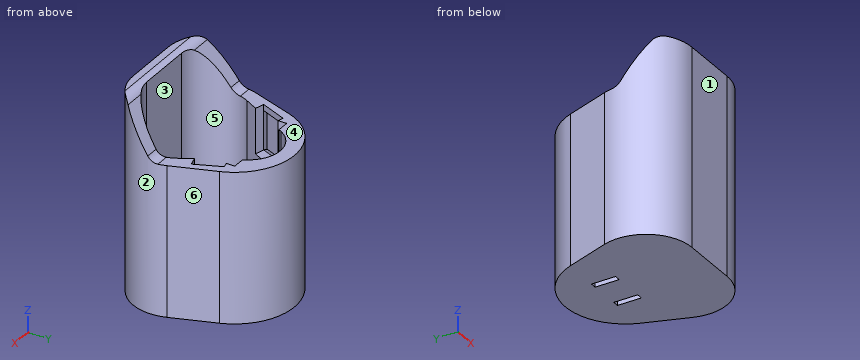
from build123d import *

# Parameters (mm, degrees)
RESSALTO_EXTRUS_O1_DEPTH   = 66
CORTE_EXTRUS_O1_DEPTH      = 53.5
CORTE_EXTRUS_O2_DEPTH      = 9.5
ESBO_O5_W                  = 2
ESBO_O5_H                  = 8
CORTE_EXTRUS_O3_DEPTH      = 72.859720289
CORTE_EXTRUS_O4_DEPTH      = 75.503821379
CORTE_EXTRUS_O4_DEPTH_BACK = 75.503821379
CORTE_EXTRUS_O6_DEPTH      = 15
ESBO_O10_W                 = 13
ESBO_O10_H                 = 9.498093923
CORTE_EXTRUS_O7_DEPTH      = 1.8
CORTE_EXTRUS_O7_DRAFT      = 23
ESBO_O11_W                 = 13
ESBO_O11_H                 = 9.498093923
CORTE_EXTRUS_O8_DEPTH      = 1.8
CORTE_EXTRUS_O8_DRAFT      = 23
FILETE10_START             = -24.75
FILETE10_DEPTH             = 49.5
FILETE11_R                 = 4
FILETE12_R                 = 4
CORTE_EXTRUS_O9_DEPTH      = 47


with BuildPart() as part:
    # Esboço2 → Ressalto-extrusão1 (new body)
    with BuildSketch(Plane.XY):
        with BuildLine():
            Line((18.875125561, 10.742838653), (23.89228324, -3.577710527))
            ThreePointArc((23.89228324, -3.577710527), (21.938999447, -17.442346217), (9.5, -23.87))
            Line((9.5, -23.87), (-9.5, -23.87))
            ThreePointArc((-9.5, -23.87), (-21.938999447, -17.442346217), (-23.89228324, -3.577710527))
            Line((-23.89228324, -3.577710527), (-18.875125561, 10.742838653))
            ThreePointArc((-18.875125561, 10.742838653), (0, 24.13), (18.875125561, 10.742838653))
        make_face()
    extrude(amount=RESSALTO_EXTRUS_O1_DEPTH)

    # Esboço3 → Corte-extrusão1 (cut)
    with BuildSketch(Plane.XY.offset(66)):
        with BuildLine():
            Line((-9.315367954, 13.892017036), (-18.902836198, -3.409513321))
            ThreePointArc((-18.902836198, -3.409513321), (-18.762160434, -14.076636702), (-9.5, -19.37))
            Line((-9.5, -19.37), (9.5, -19.37))
            ThreePointArc((9.5, -19.37), (18.762160434, -14.076636702), (18.902836198, -3.409513321))
            Line((18.902836198, -3.409513321), (9.315367954, 13.892017036))
            ThreePointArc((9.315367954, 13.892017036), (0, 19.38), (-9.315367954, 13.892017036))
        make_face()
    extrude(amount=-CORTE_EXTRUS_O1_DEPTH, mode=Mode.SUBTRACT)

    # Esboço4 → Corte-extrusão2 (cut)
    with BuildSketch(Plane.XY.offset(12.5)):
        with BuildLine():
            Line((-9.315367954, 13.892017036), (-18.88094029, -3.37))
            Line((-18.88094029, -3.37), (18.88094029, -3.37))
            Line((18.88094029, -3.37), (9.315367954, 13.892017036))
            ThreePointArc((9.315367954, 13.892017036), (0, 19.38), (-9.315367954, 13.892017036))
        make_face()
    extrude(amount=-CORTE_EXTRUS_O2_DEPTH, mode=Mode.SUBTRACT)

    # Esboço5 → Corte-extrusão3 (cut, through all)
    with BuildSketch(Plane.XY.offset(3)):
        with Locations((-6, 7.13)):
            Rectangle(ESBO_O5_W, ESBO_O5_H)
        with Locations((6, 7.13)):
            Rectangle(ESBO_O5_W, ESBO_O5_H)
    extrude(amount=-CORTE_EXTRUS_O3_DEPTH, mode=Mode.SUBTRACT)

    # Esboço6 → Corte-extrusão4 (cut, two sides: drawn at the far end of the back side and taken through both)
    with BuildSketch(Plane(origin=(0, 0, 0), x_dir=(0, 0, -1), z_dir=(1, 0, 0)).offset(-CORTE_EXTRUS_O4_DEPTH_BACK)):
        Polygon((-73.252948894, -8.37), (-72.738467135, 18.869608141), (-69.396784042, 24.687681426), (-65.169347817, 25.830591912), (-50, 27.529066054), (-50, -8.37), (-66, -19.37), (-66, -23.87), (-79.476934269, -23.87), (-79.476934269, -8.37), align=None)
    extrude(amount=CORTE_EXTRUS_O4_DEPTH + CORTE_EXTRUS_O4_DEPTH_BACK, mode=Mode.SUBTRACT)

    # Esboço7 → Corte-extrusão6 (cut)
    with BuildSketch(Plane.XY.offset(50)):
        Polygon((0, -3.37), (19.549187838, 1.7499651), (15.86238212, 10.5033217), (2e-09, 6.348937203), (-15.862382121, 10.5033217), (-19.549187841, 1.7499651), align=None)
    extrude(amount=-CORTE_EXTRUS_O6_DEPTH, mode=Mode.SUBTRACT)


with BuildPart() as corte_extrus_o7_tool:
    # Esboço10 → Corte-extrusão7 (with draft: the straight prism first)
    with BuildSketch(Plane(origin=(17.229716404, 7.256943806, 0), x_dir=(0, 0, 1), z_dir=(-0.9215908655875538, -0.3881626932944273, 0))):
        with Locations((41.5, -1.226466591)):
            Rectangle(ESBO_O10_W, ESBO_O10_H)
    extrude(amount=-CORTE_EXTRUS_O7_DEPTH)
    # Corte-extrusão7: the draft: its side faces are tilted about the plane it starts from
    corte_extrus_o7_sides = [corte_extrus_o7_tool.faces().sort_by_distance(p)[0] for p in [
        (16.691813899, 10.852668124, 41.5),
        (18.535216758, 6.475989824, 35),
        (20.378619617, 2.099311524, 41.5),
        (18.535216758, 6.475989824, 48),
    ]]
    draft(corte_extrus_o7_sides, Plane(origin=(17.229716404, 7.256943806, 0), x_dir=(0, 0, 1), z_dir=(-0.9215908655875538, -0.3881626932944273, 0)), CORTE_EXTRUS_O7_DRAFT)


with BuildPart() as part_1:
    add(part.part)

    # Corte-extrusão7: cut by corte_extrus_o7_tool
    add(corte_extrus_o7_tool.part, mode=Mode.SUBTRACT)


with BuildPart() as corte_extrus_o8_tool:
    # Esboço11 → Corte-extrusão8 (with draft: the straight prism first)
    with BuildSketch(Plane(origin=(-17.229716404, 7.256943809, 0), x_dir=(0, 0, -1), z_dir=(0.9215908655337633, -0.3881626934221387, 0))):
        with Locations((-41.5, -1.226466593)):
            Rectangle(ESBO_O11_W, ESBO_O11_H)
    extrude(amount=-CORTE_EXTRUS_O8_DEPTH)
    # Corte-extrusão8: the draft: its side faces are tilted about the plane it starts from
    corte_extrus_o8_sides = [corte_extrus_o8_tool.faces().sort_by_distance(p)[0] for p in [
        (-18.53521676, 6.475989824, 48),
        (-20.37861962, 2.099311524, 41.5),
        (-18.53521676, 6.475989824, 35),
        (-16.6918139, 10.852668124, 41.5),
    ]]
    draft(corte_extrus_o8_sides, Plane(origin=(-17.229716404, 7.256943809, 0), x_dir=(0, 0, -1), z_dir=(0.9215908655337633, -0.3881626934221387, 0)), CORTE_EXTRUS_O8_DRAFT)


with BuildPart() as part_2:
    add(part_1.part)

    # Corte-extrusão8: cut by corte_extrus_o8_tool
    add(corte_extrus_o8_tool.part, mode=Mode.SUBTRACT)

    # Filete10: read off the stored shape, not the designer's step
    # Filete10 outline → Filete10 (cut)
    with BuildSketch(Plane.YZ.offset(FILETE10_START)):
        with BuildLine():
            ThreePointArc((-21.47412196, 66), (-19.611926245, 65.540088576), (-18.177953073, 64.266113561))
            Line((-18.177953073, 64.266113561), (-19.37, 66))
            Line((-19.37, 66), (-21.47412196, 66))
        make_face()
    extrude(amount=FILETE10_DEPTH, mode=Mode.SUBTRACT)

    # Filete11
    filete11_edges = [part_2.edges().sort_by_distance(p)[0] for p in [
        (-22.497521656, -8.37, 50),
    ]]
    fillet(filete11_edges, radius=FILETE11_R)

    # Filete12
    filete12_edges = [part_2.edges().sort_by_distance(p)[0] for p in [
        (22.497521656, -8.37, 50),
    ]]
    fillet(filete12_edges, radius=FILETE12_R)

    # Esboço12 → Corte-extrusão9 (cut)
    with BuildSketch(Plane.XY.offset(50)):
        Polygon((14, 12.88), (14, 7.88), (-14, 7.88), (-14, 12.88), (0, 12.88), align=None)
    extrude(amount=-CORTE_EXTRUS_O9_DEPTH, mode=Mode.SUBTRACT)


solid = part_2.part
CAD build for the part. Positions are in the model's coordinates, mm. Face numbers are marked on the shaded views. A direction names the side the tool comes from. Give positions to 0.01 mm unless a question says otherwise; leave off trailing zeros. Write each loop counter-clockwise with the first axis right and the second up, starting at its lowest first coordinate (ties: lowest second). Pieces come first, ordered by that corner, then holes. Notation, with made-up numbers: (74, 87) -> (100, 87) arc R31 ccw to (100, 117) -> close; hole circle Ø5 at (-26.5, 19.5). An arc over 180 degrees is marked (long way). Return JSON: item names as keys, results as strings.
Item 1: Drop flat-ended pins along their axis: pin 1 (5 mm diameter, centred on x = -5, z = 6.5, fed in from +Y); pin 2 (2 mm diameter, centred on x = -18, y = 5.5, fed in from +Z); pin 3 (12 mm diameter, centred on x = -10, z = 28, fed in from +Y). Give the stop position or say it passes through.
Answer below:
{"pin 1": "stops at y = 23.97", "pin 2": "stops at z = 50", "pin 3": "stops at y = 23.73"}
Item 2: Two-plate mould, pull along Y, no slides. Class the marked faces 1, 2 and 3: +Y half, -Y half, draft (parallel to the pull), parting line (faces both ways), or undercut.
Answer below:
{"face 1": "-Y half", "face 2": "parting line", "face 3": "undercut"}
Item 3: Drill centre lines: probe 1 along Z at (x, y) = (-13.5, 6); probe 2 along Y at (x, z) = (-17, 35.5); probe 3 along Z at (x, y) = (22, -2). Where is each one in solid material? Low to high.
Answer below:
{"probe 1": "z = 0 to 3", "probe 2": "y = -21.9 to -16.32, 0.02 to 1.08, 11.67 to 14.67", "probe 3": "z = 0 to 50"}
Item 4: Band-saw the part on B-B (y = 4.5). List the corners of the cut face in (x, z), then the cut area to 3 significant figures.
Answer below:
{"outline": "(-21.06, 0) -> (-7, 0) -> (-7, 3) -> (-14.52, 3) -> (-14.52, 35) -> (-18.39, 35) -> (-20.34, 34.24) -> (-20.34, 48.76) -> (-18.39, 48) -> (-18.39, 50) -> (-21.06, 50) -> close; (-5, 0) -> (5, 0) -> (5, 3) -> (-5, 3) -> close; (7, 0) -> (21.06, 0) -> (21.06, 50) -> (18.39, 50) -> (18.39, 48) -> (20.34, 48.76) -> (20.34, 34.24) -> (18.39, 35) -> (14.52, 35) -> (14.52, 3) -> (7, 3) -> close", "area": "559 mm2"}
Item 5: Band-saw the part on C-C (z = 21). List the corners of the cut face in (x, y), then the cut area to 3 significant figures.
Answer below:
{"outline": "(-23.89, -3.58) arc R15.25 ccw to (-9.5, -23.87) -> (9.5, -23.87) arc R15.25 ccw to (23.89, -3.58) -> (18.88, 10.74) arc R20 ccw to (-18.88, 10.74) -> close; hole (-18.9, -3.41) arc R10.75 ccw to (-9.5, -19.37) -> (9.5, -19.37) arc R10.75 ccw to (18.9, -3.41) -> (12.65, 7.88) -> (14, 7.88) -> (14, 12.88) -> (9.88, 12.88) -> (9.32, 13.89) arc R10.65 ccw to (-9.32, 13.89) -> (-9.88, 12.88) -> (-14, 12.88) -> (-14, 7.88) -> (-12.65, 7.88) -> close", "area": "702 mm2"}
Item 6: Band-saw the part on A-A (z = 41.5). List the corners of the cut face in (x, y).
Answer below:
{"outline": "(-23.89, -3.58) arc R15.25 ccw to (-9.5, -23.87) -> (9.5, -23.87) arc R15.25 ccw to (23.89, -3.58) -> (18.88, 10.74) arc R20 ccw to (-18.88, 10.74) -> close; hole (-21.5, 1.74) -> (-19.55, 1.75) -> (-16.49, 0.95) -> (-18.9, -3.41) arc R10.75 ccw to (-9.5, -19.37) -> (9.5, -19.37) arc R10.75 ccw to (18.9, -3.41) -> (16.49, 0.95) -> (19.55, 1.75) -> (21.5, 1.74) -> (17.22, 11.91) -> (15.86, 10.5) -> (14, 10.02) -> (14, 12.88) -> (9.88, 12.88) -> (9.32, 13.89) arc R10.65 ccw to (-9.32, 13.89) -> (-9.88, 12.88) -> (-14, 12.88) -> (-14, 10.02) -> (-15.86, 10.5) -> (-17.22, 11.91) -> close"}
Item 7: Band-saw the part on D-D (z = 60). List the corners of the cut face in (x, y) (3 decimals), then the cut area to 3 significant figures.
Answer below:
{"outline": "(-23.236, -15.245) arc R15.25 ccw to (-9.5, -23.87) -> (9.5, -23.87) arc R15.25 ccw to (23.236, -15.245) -> (17.966, -15.245) arc R10.75 cw to (9.5, -19.37) -> (-9.5, -19.37) arc R10.75 cw to (-17.966, -15.245) -> close", "area": "207 mm2"}
Item 8: Tool access for the marked faces 4, 5 and 6: list every direction of +Z, -Z, +X, -X, +Y, -Y with a clear straight run to the whole face (end or side of a thin tool).
Answer below:
{"face 4": "+Z, +X, -X, +Y", "face 5": "+Z", "face 6": "+Z, -Z, +X, +Y"}
